Part model, mm, in its own coordinate system. Give positions to 0.01 mm unless a question says otherwise; leave off trailing zeros. Write each loop counter-clockwise with the first axis right and the second up, starting at its lowest first coordinate (ties: lowest second). Pieces come first, ordered by that corner, then holes. Notation, with made-up numbers: M 75.25,75 L 108.25,75 A36 cw 108.25,110 Z; hole C 12.5,-25 d7. An arc over 180 degrees is marked long. Answer as CSV lines item,"result". Start each with the question number.
Item 1: Wall check: L1, parallel to Z at x = 93.5, y = 0.5; L2, parallel to Z at x = 104, y = -0.25. Give the ranges that are in metal, low to high. Write a range as from..to.
Item 2: Pin check, flat tips, straight feed: pin 1 (1.5 mm diameter, centred on x = 90.5, y = -0.5, fed in from -Z); pin 2 (2 mm diameter, centred on x = 83.5, z = -2.5, fed in from +Y); pin 3 (1.5 mm diameter, centred on x = 116, z = -1, fed in from -Y). Stop position of each tip, or through.
Item 3: Band-saw the part on A-A, the plane x = 173.5. List the corners of the cut face in (y, z).
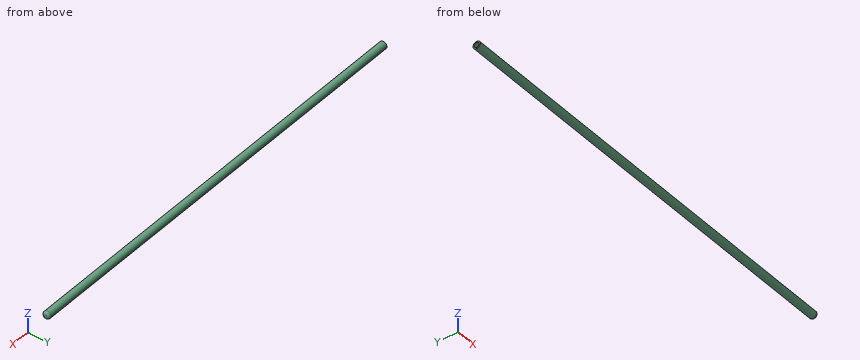
from build123d import *

# Parameters (mm, degrees)
F0_R     = 3
F0_R_2   = 2
F1_DEPTH = 350
F2_R     = 3.0183078128
F3_DEPTH = 2
F4_R     = 1.99999


# Not quite as in the source:
# - a fillet or chamfer is up to 0.001 mm smaller than in the source, because OpenCascade refuses the exact size


with BuildPart() as f1:
    # F0 (on Right) → F1 (new body)
    with BuildSketch(Plane.YZ):
        Circle(F0_R)
        Circle(F0_R_2, mode=Mode.SUBTRACT)
    extrude(amount=F1_DEPTH)

    # F2 (on face) → F3 (join)
    with BuildSketch(Plane.YZ.offset(350)):
        Circle(F2_R)
    extrude(amount=F3_DEPTH)

    # F4 (radius 2 in the source; OpenCascade refuses exactly that, so slightly less here)
    f4_edges = [f1.edges().sort_by_distance(p)[0] for p in [
        (352, -3.018308, 0),
    ]]
    fillet(f4_edges, radius=F4_R)


solid = f1.part
Output:
1,L1,"-2.96..-1.94, 1.94..2.96"
1,L2,"-2.99..-1.98, 1.98..2.99"
2,pin 1,"z = -3"
2,pin 2,"y = 2.6"
2,pin 3,"y = -2.99"
3,outline,"C 0,0 d6; hole C 0,0 d4"
